```python
from build123d import *

# Parameters (mm, degrees)
EXTRUDE_1_DEPTH     = 150
CUT_EXTRUDE_1_DEPTH = 309.196154086
CUT_EXTRUDE_3_REACH = 4
SKETCH_3_W          = 150
SKETCH_3_H          = 270.46


with BuildPart() as part:
    # 草图1 → 凸台-拉伸1 (new body)
    with BuildSketch(Plane(origin=(0, 0, 0), x_dir=(0, 0, -1), z_dir=(1, 0, 0))):
        Polygon((0, 0), (-34, -280), (276.46, -280), (242.46, 0), align=None)
        Polygon((240.688166201, -2), (1.771833799, -2), (-31.742451915, -278), (274.202451915, -278), align=None, mode=Mode.SUBTRACT)
    extrude(amount=EXTRUDE_1_DEPTH)

    # 草图2 → 切除-拉伸1 (cut, through all)
    with BuildSketch(Plane(origin=(0, 0, 0), x_dir=(1, 0, 0), z_dir=(0, 0.120543125, 0.992708091))):
        Polygon((0, 0), (0, -282.056731882), (60, -282.056731882), align=None)
    extrude(amount=-CUT_EXTRUDE_1_DEPTH, mode=Mode.SUBTRACT)

    # 草图3 → 切除-拉伸3 (cut, up to next)
    with BuildSketch(Plane(origin=(0, -278, 0), x_dir=(1, 0, 0), z_dir=(0, 1, 0)), mode=Mode.PRIVATE) as cut_extrude_3_sk1:
        with Locations((75, 121.23)):
            Rectangle(SKETCH_3_W, SKETCH_3_H)
    cut_extrude_3_tool1 = extrude(cut_extrude_3_sk1.sketch, amount=-CUT_EXTRUDE_3_REACH, mode=Mode.PRIVATE) & part.part
    add(cut_extrude_3_tool1.solids().sort_by_distance((75, -278, -121.23))[0], mode=Mode.SUBTRACT)


solid = part.part
```
Verification items for the finished model (mm, model axes). A direction names the side the tool comes from. Give positions to 0.01 mm unless a question says otherwise; leave off trailing zeros. Loops run counter-clockwise (first coordinate to the right, second up) from the corner with the lowest first, then second, coordinate; pieces in that order, holes last. Notation, with made-up numbers: M -12,53 L 31,53 A15 cw 31,68 Z; hole C 17.25,-6.75 d9. An arc over 180 degrees is marked long. Return JSON: item names as keys, results as strings.
1) Tool access check on faces 5 (the flat face through (90.62, -138.04, 16.76)), 6 (the flat face through (74, -2, -123)), 7 (the flat face through (104, -278, 23)). Record the directions out of +Z, -Z, +X, -X, +Y, -Y that give a thin tool (end or side, any length) a straight path to the whole face; none if there is none.
Findings:
{"face 5": "+Z, +X, -X, +Y", "face 6": "+X, -X, -Y", "face 7": "+X, -X"}
2) Section check A-A, the plane y = -100. Enter the section's corners in (x, z), and give its area (3 significant figures).
Findings:
{"outline": "M 14.59,-254.6 L 150,-254.6 L 150,-252.59 L 14.64,-252.59 Z; M 21.38,10.13 L 150,10.13 L 150,12.14 L 21.43,12.14 Z", "area": "532 mm2"}
3) Material ranges on L1, parallel to Z at x = 76, y = -16.5; L2, parallel to Y at x = 124, z = -208.5; L3, parallel to Z at x = 81.5, y = -88, recorded low to high. Write a range as [from, to].
Findings:
{"L1": "z = [-244.46, -242.45], [-0.01, 2]", "L2": "y = [-2, 0]", "L3": "z = [-253.15, -251.13], [8.67, 10.69]"}
4) Mould release check, pull along Y, two halves, no side actions. Record for faces 1 (the flat face through (104, -280, 24)), 2 (the flat face through (90.62, -141.93, -257.68)), 3 (the flat face through (90.62, -141.96, -259.7)), 4 (the flat face through (0, -1.6, -131.6)): released by +Y, released by -Y, zero draft, split by the parting line, or undercut.
Findings:
{"face 1": "released by -Y", "face 2": "undercut", "face 3": "released by +Y", "face 4": "zero draft"}
5) Section check B-B, the plane x = 70. Enter the section's corners in (y, z).
Findings:
{"outline": "M -280,-276.46 L 0,-242.46 L 0,0 L -280,34 L -280,14 L -278,14 L -278,31.74 L -2,-1.77 L -2,-240.69 L -278,-274.2 L -278,-256.46 L -280,-256.46 Z"}
6) Section check D-D, the plane y = -54.5. Enter the section's corners in (x, z), and give its area (3 significant figures).
Findings:
{"outline": "M 5.12,-249.08 L 150,-249.08 L 150,-247.06 L 5.17,-247.06 Z; M 11.63,4.6 L 150,4.6 L 150,6.62 L 11.68,6.62 Z", "area": "571 mm2"}
7) Gauge pin test, flat ends, axial feed: P1, Ø2, axis at x = 47.5, y = -88, coming from the -Z side; P2, Ø4, axis at x = 20, y = -109.5, coming from the -Z side; P3, Ø3, axis at x = 66.5, z = -163.5, coming from the -Y side. Record the tip position at first contact, or that the pin passes through.
Findings:
{"P1": "stops at z = -253.27", "P2": "stops at z = -256", "P3": "stops at y = -2"}
8) Section check C-C, the plane z = -142. Enter the section's corners in (x, y).
Findings:
{"outline": "M 0,-2 L 150,-2 L 150,0 L 0,0 Z"}
